For this review, use the dimensioned drawing (mm, ordinates from the lowest corner) and the shaded views. A direction names the side the tool comes from. Give positions to 0.01 mm unless a question says otherwise; leave off trailing zeros. Order: outer loops, then holes, each group sorted by start corner. A loop starts at its lowest first (then second) coordinate and runs counter-clockwise, first axis right, second up. Notation, with made-up numbers: (66.25, 37.5) - (125.25, 37.5) arc R22 cw to (125.25, 69.5) - close; hole circle Ø10 at (-38, 86.5). An arc over 180 degrees is marked (long way). One line per item, written item: value.
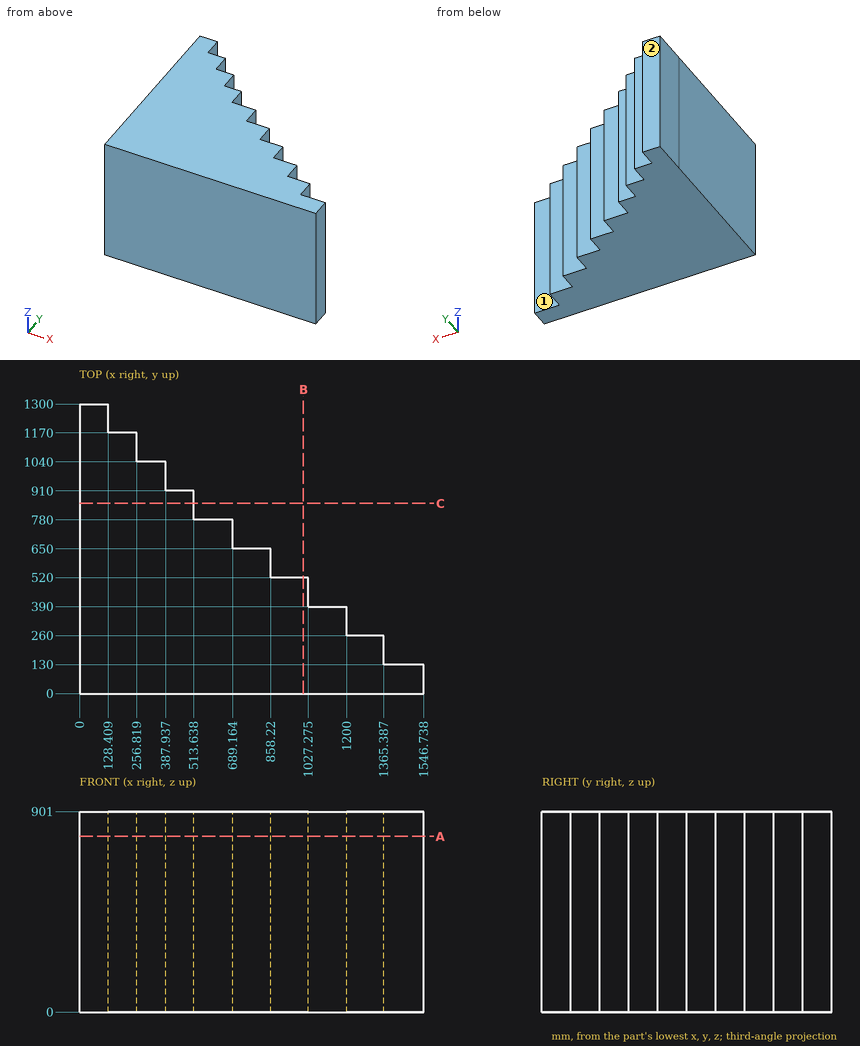
(1) For P1, Ø6, axis at y = 920.5, z = 307, coming from the +X side; P2, Ø10, axis at x = 1321, z = 768, coming from the +Y side; P3, Ø5, axis at y = 1067.5, z = 459, coming from the +X side, all flat-tipped, find the tip position at first contact; note any pin that passes through.
Answers below:
P1: stops at x = 387.94
P2: stops at y = 260
P3: stops at x = 256.82
(2) Take a section at B-B (x = 1005). Write out the cut boundary in (y, z).
Answers below:
outline: (0, 0) - (520, 0) - (520, 901) - (0, 901) - close
(3) Machinability: for the marked faces 1 and 2, which of the approach directions +Z, -Z, +X, -X, +Y, -Y give a long, thin tool a straight path to every point of the face, cutting with its end or side? Answer none if there is none.
Answers below:
face 1: +Z, -Z, +X, +Y
face 2: +Z, -Z, +X, -X, +Y
(4) Take a section at C-C (y = 853.5). Write out the cut boundary in (x, z), then the cut area to 3 significant figures.
Answers below:
outline: (0, 0) - (513.64, 0) - (513.64, 901) - (0, 901) - close
area: 463,000 mm^2
(5) Wall thickness on line 1 (Y direction, x = 867.5, z = 632); line 2 (Y direction, x = 794, z = 740.5); line 3 (X direction, y = 980.5, z = 388): over which ranges is each line inside the solid? List them lowest first. Write a range as from..to.
Answers below:
line 1: y = 0..520
line 2: y = 0..650
line 3: x = 0..387.94
(6) Take a section at A-A (z = 789.5). Write out the cut boundary in (x, y) (1 decimal).
Answers below:
outline: (0, 0) - (1546.7, 0) - (1546.7, 130) - (1365.4, 130) - (1365.4, 260) - (1200, 260) - (1200, 390) - (1027.3, 390) - (1027.3, 520) - (858.2, 520) - (858.2, 650) - (689.2, 650) - (689.2, 780) - (513.6, 780) - (513.6, 910) - (387.9, 910) - (387.9, 1040) - (256.8, 1040) - (256.8, 1170) - (128.4, 1170) - (128.4, 1300) - (0, 1300) - close
